For this review, take the finished solid that the model builds, in its own axes (mm). Coordinates: 2 decimals unless noted, no trailing zeros. Order: outer loops, then holes, each group sorted by start corner. A loop starts at its lowest first (then second) coordinate and runs counter-clockwise, first axis right, second up. Notation, with made-up numbers: (65.25, 57) -> (100.25, 57) arc R32 ccw to (100.25, 94) -> close; hole circle Ø3 at (59.25, -24.5). An arc over 180 degrees is marked (long way). Write item = value, one per line. Start each with the question number.
1) Consider section C-C on x = 11.25. Give the boundary of the cut face in (y, z).
2) Wall thickness on probe 1 along Y at (x, z) = (0.05, 0); probe 2 along X at (y, z) = (-0.4, 0.8); probe 3 along Y at (x, z) = (4, -0.1): over which ranges is each line inside the solid? List them lowest first. Write a range as [from, to].
3) Insertion check: pin 1 Ø1 at (x, z) = (2, -1) entering from -Y. The pin has a flat end and moves straight along its axis. Give the tip position at first contact, or say it passes through.
4) Draft analysis for pull direction Y (two halves, no side actions). For faces 1 (the face through (0.16, 0, 0)), 2 (the face through (13.66, 0, 0)), 3 (the face through (6.66, -0.45, 1.43)), state which applies: +Y half, -Y half, draft (parallel to the pull), parting line (faces both ways), or undercut.
5) Consider section A-A on z = 0. Give the boundary of the cut face in (x, y).
from build123d import *

# Parameters (mm, degrees)
ESQUISSE1_W             = 14
ESQUISSE1_H             = 1.5
CONG_1_R                = 0.2
ESQUISSE2_R             = 1.25
ENL_V_MAT_EXTRU_1_DEPTH = 0.5


with BuildPart() as part:
    # Esquisse1 → Révolution1 (revolve)
    with BuildSketch(Plane.XY, mode=Mode.PRIVATE) as r_volution1_sk:
        with Locations((6.66, 0.75)):
            Rectangle(ESQUISSE1_W, ESQUISSE1_H)
    revolve(r_volution1_sk.sketch.rotate(Axis((-5.768945874, 0, 0), (1, 0, 0)), 90), axis=Axis((-5.768945874, 0, 0), (1, 0, 0)))

    # Congé1
    cong_1_edges = [part.edges().sort_by_distance(p)[0] for p in [
        (13.66, 0, -1.5),
    ]]
    fillet(cong_1_edges, radius=CONG_1_R)

    # Esquisse2 → Enlèv. mat.-Extru.1 (cut)
    with BuildSketch(Plane.ZY.offset(0.34)):
        Circle(ESQUISSE2_R)
    extrude(amount=-ENL_V_MAT_EXTRU_1_DEPTH, mode=Mode.SUBTRACT)


solid = part.part
Answer sheet:
q1.outline = circle Ø3 at (0, 0)
q2.probe_1 = [-1.5, -1.25], [1.25, 1.5]
q2.probe_2 = [0.16, 13.66]
q2.probe_3 = [-1.5, 1.5]
q3.pin_1 = -1.41
q4.face_1 = undercut
q4.face_2 = draft
q4.face_3 = parting line
q5.outline = (-0.34, -1.5) -> (13.46, -1.5) arc R0.2 ccw to (13.66, -1.3) -> (13.66, 1.3) arc R0.2 ccw to (13.46, 1.5) -> (-0.34, 1.5) -> (-0.34, 1.25) -> (0.16, 1.25) -> (0.16, -1.25) -> (-0.34, -1.25) -> close
